from build123d import *
from build123d.topology import SkipClean

# Parameters (mm, degrees)
BOSS_EXTRUDE1_DEPTH = 23
BOSS_EXTRUDE2_DEPTH = 2
SKETCH3_R           = 1.05
BOSS_EXTRUDE3_DEPTH = 14.5
CUT_EXTRUDE1_REACH  = 90.03
SKETCH4_W           = 17
SKETCH4_H           = 23.2
CUT_EXTRUDE2_DEPTH  = 7
SKETCH6_R           = 1.05
CUT_EXTRUDE3_DEPTH  = 61.135264197
SKETCH7_W           = 18
SKETCH7_H           = 33
CUT_EXTRUDE4_DEPTH  = 51.162236792
FILLET1_R           = 2
SKETCH8_R           = 2
CUT_EXTRUDE5_DEPTH  = 1.4


with BuildPart() as part:
    # Sketch1 → Boss-Extrude1 (new, symmetric)
    with BuildSketch(Plane.XY):
        with BuildLine():
            Line((0, 41), (3.464101615, 39))
            Line((3.464101615, 39), (7.687881875, 39))
            ThreePointArc((7.687881875, 39), (19.943980289, 22.03249582), (10.356028111, 3.42660107))
            Line((10.356028111, 3.42660107), (0, 3.42660107))
            Line((0, 3.42660107), (0, 0))
            Line((0, 0), (10.356028111, 0))
            ThreePointArc((10.356028111, 0), (22.999858198, 20.45585385), (10.5, 41))
            Line((10.5, 41), (0, 41))
        make_face()
    extrude(amount=BOSS_EXTRUDE1_DEPTH, both=True)

    # Sketch2 → Boss-Extrude2 (add)
    with BuildSketch(Plane.XY.offset(23)):
        with BuildLine():
            Line((0, 41), (0, 3.42660107))
            Line((0, 3.42660107), (10.356028111, 3.42660107))
            ThreePointArc((10.356028111, 3.42660107), (19.943980289, 22.03249582), (7.687881875, 39))
            Line((7.687881875, 39), (3.464101615, 39))
            Line((3.464101615, 39), (0, 41))
        make_face()
    boss_extrude2 = extrude(amount=-BOSS_EXTRUDE2_DEPTH)

    # Sketch3 → Boss-Extrude3 (add, symmetric)
    with BuildSketch(Plane.XY):
        Polygon((12.5, -40.8), (6.5, -40.8), (6.5, -35.8), (12.5, -35.8), (12.5, -1.8), (6.5, -1.8), (6.5, 3.2), (12.5, 3.2), (17.5, 3.2), (17.5, -40.8), align=None)
        with Locations((9, 0.7)):
            Circle(SKETCH3_R, mode=Mode.SUBTRACT)
        with Locations(Location((9, -38.3, 0), (0, 0, 180))):
            Circle(SKETCH3_R, mode=Mode.SUBTRACT)
    extrude(amount=BOSS_EXTRUDE3_DEPTH, both=True)

    # Mirror2: Boss-Extrude2 across plane
    add(boss_extrude2.mirror(Plane.XY))

    # Cut-Extrude1: up to this face of the body (flat: up to its plane)
    cut_extrude1_end = Plane(part.part.faces().sort_by_distance((5.178014055, 3.42660107, 0))[0])
    # Sketch4 → Cut-Extrude1 (cut, up to the picked face)
    with BuildSketch(Plane.XZ.offset(40.8), mode=Mode.PRIVATE) as cut_extrude1_sk1:
        with Locations((4, 0)):
            Rectangle(SKETCH4_W, SKETCH4_H)
    cut_extrude1_tool1 = split(extrude(cut_extrude1_sk1.sketch, amount=-CUT_EXTRUDE1_REACH, mode=Mode.PRIVATE), bisect_by=cut_extrude1_end, keep=Keep.BOTH, mode=Mode.PRIVATE)
    add(cut_extrude1_tool1.solids().sort_by(Axis((4, -40.8, 0), (0, 1, 0)))[0], mode=Mode.SUBTRACT)

    # Sketch5 → Cut-Extrude2 (cut)
    with BuildSketch(Plane.XZ):
        Polygon((0, -11.6), (6.5, -11.6), (6.5, -14.5), (10.356028111, -14.5), (10.356028111, -23), (0, -23), align=None)
        Polygon((6.5, 11.6), (0, 11.6), (0, 23), (10.356028111, 23), (10.356028111, 14.5), (6.5, 14.5), align=None)
    extrude(amount=-CUT_EXTRUDE2_DEPTH, mode=Mode.SUBTRACT)

    # Sketch6 → Cut-Extrude3 (cut, through all)
    with SkipClean():  # the faces are left unmerged after this step: merging them gives an invalid solid
        with BuildSketch(Plane.XY.offset(14.5)):
            with Locations(Location((9, 0.7, 0), (0, 0, 180))):
                Circle(SKETCH6_R)
        extrude(amount=-CUT_EXTRUDE3_DEPTH, mode=Mode.SUBTRACT)

    # Sketch7 → Cut-Extrude4 (cut, through all)
    with SkipClean():  # the faces are left unmerged after this step: merging them gives an invalid solid
        with BuildSketch(Plane(origin=(17.5, 0, 0), x_dir=(0, 0, -1), z_dir=(1, 0, 0))):
            with Locations((0, -18.8)):
                Rectangle(SKETCH7_W, SKETCH7_H)
        extrude(amount=-CUT_EXTRUDE4_DEPTH, mode=Mode.SUBTRACT)

    # Fillet1
    fillet1_edges = [part.edges().sort_by_distance(p)[0] for p in [
        (6.5, -40.8, -13.05),
        (6.5, -35.8, -13.05),
        (6.5, -1.8, -13.05),
        (6.5, 3.42660107, -13.05),
        (6.5, 3.42660107, 13.05),
        (15, -35.3, -9),
        (15, -35.3, 9),
        (15, -2.3, 9),
        (15, -2.3, -9),
        (17.5, -40.8, 0),
        (6.5, -1.8, 13.05),
        (6.5, -35.8, 13.05),
        (6.5, -40.8, 13.05),
    ]]
    fillet(fillet1_edges, radius=FILLET1_R)

    # Sketch8 → Cut-Extrude5 (cut)
    with SkipClean():  # the faces are left unmerged after this step: merging them gives an invalid solid
        with BuildSketch(Plane.XY.offset(14.5)):
            with Locations((9, 0.7)):
                Circle(SKETCH8_R)
            with Locations((9, -38.3)):
                Circle(SKETCH8_R)
        cut_extrude5 = extrude(amount=-CUT_EXTRUDE5_DEPTH, mode=Mode.SUBTRACT)

    # Mirror3: Cut-Extrude5 across plane
    with SkipClean():  # the faces are left unmerged after this step: merging them gives an invalid solid
        add(cut_extrude5.mirror(Plane.XY), mode=Mode.SUBTRACT)


solid = part.part
Design review of the part built by this model. Coordinates are the model's own, in mm. A direction names the side the tool comes from. Give positions to 0.01 mm unless a question says otherwise; leave off trailing zeros. Loops run counter-clockwise (first coordinate to the right, second up) from the corner with the lowest first, then second, coordinate; pieces in that order, holes last. Notation, with made-up numbers: (77, 89.25) - (93, 89.25) arc R19 ccw to (93, 118.25) - close; hole circle Ø6 at (75, -3.5). An arc over 180 degrees is marked (long way). Use CSV: the item, a comma, the result in double quotes. Start each with the question number.
1. Machinability: for faces 1 (the flat face through (9, 3.427, 13)), 2 (the flat face through (5, 7, 22)), 3 (the flat face through (12.5, -19, 9.5)), 4 (the cylindrical face through (14.96, -34.7, 8.43)), which of the approach directions +Z, -Z, +X, -X, +Y, -Y give a long, thin tool a straight path to every point of the face, cutting with its end or side? Answer none if there is none.
2. Wall thickness on L1, parallel to Z at x = 16, y = 26; L2, parallel to Z at x = 15.75, y = -18; L3, parallel to Y at x = 9, z = 13.5: over which ranges is each line inside the solid? List them lowest first.
3. Insertion check: P1, Ø3.5, axis at x = 12, y = -9.5, coming from the -Z side; P2, Ø23, axis at y = -20, z = 4, coming from the -X side; P3, Ø2, axis at x = 3, z = 22, coming from the -Y side; P4, Ø12, axis at x = 4, y = -13, coming from the +Z side. Each pin has a flat end and moves straight along its axis. Give the tip position at first contact, or say it passes through.
4. Add section C-C (z = -20). State the section outline as (x, y) points.
5. Draft analysis for pull direction Y (two halves, no side actions). For faces 5 (the cylindrical face through (7.1, -40.23, 13.03)), 6 (the flat face through (15, -19, 9)), 7 (the flat face through (10, -35.8, -13)), 8 (the flat face through (10.1, 1.4, -11.6)), state which applies: released by +Y, released by -Y, zero draft, split by the parting line, or undercut.
6. Add section D-D (y = 31.5). State the section outline as (x, z) points, plus the area to 3 significant figures.
7. Add section B-B (y = -25). State the section outline as (x, z) points.
8. Add section A-A (z = 1.5). State the section outline as (x, y) points.
Results found:
1,face 1,"+Z, -Z, -X"
1,face 2,"+Z, -Z, -X, -Y"
1,face 3,"-X"
1,face 4,"+X, -X"
2,L1,"z = -23 to -21, 21 to 23"
2,L2,"z = -14.5 to -9, 9 to 14.5"
2,L3,"y = -40.8 to -40.3, -36.3 to -35.8, -1.8 to -1.3, 2.7 to 3.43, 38.4 to 41"
3,P1,"stops at z = -14.5"
3,P2,"stops at x = 12.5"
3,P3,"stops at y = 7"
3,P4,"passes through"
4,outline,"(0, 41) - (3.46, 39) - (7.69, 39) arc R20 cw to (10.36, 3.43) - (10.36, 0) arc R23 ccw to (10.5, 41) - close"
5,face 5,"released by -Y"
5,face 6,"undercut"
5,face 7,"undercut"
5,face 8,"zero draft"
6,outline,"(0, -23) - (20.22, -23) - (20.22, 23) - (0, 23) - (0, 21) - (16.73, 21) - (16.73, -21) - (0, -21) - close"
6,area,"228 mm²"
7,outline,"(12.5, -14.5) - (17.5, -14.5) - (17.5, -9) - (12.5, -9) - close; (12.5, 9) - (17.5, 9) - (17.5, 14.5) - (12.5, 14.5) - close"
8,outline,"(0, 41) - (3.46, 39) - (7.69, 39) arc R20 cw to (10.36, 3.43) - (12.5, 3.43) - (12.5, -2.3) - (17.5, -2.3) - (17.5, 3.2) - (15.11, 3.2) arc R23 ccw to (10.5, 41) - close; (12.5, -40.8) - (15.5, -40.8) arc R2 ccw to (17.5, -38.8) - (17.5, -35.3) - (12.5, -35.3) - close"
